Read the model definition and answer for the solid it produces. Units are mm, in the model's axes. Face numbers are marked on the shaded views. A direction names the side the tool comes from. Give positions to 0.01 mm unless a question says otherwise; leave off trailing zeros. Order: outer loops, then holes, each group sorted by start corner. A loop starts at its lowest first (then second) coordinate and runs counter-clockwise, first axis right, second up. Notation, with made-up numbers: (55, -5) - (88, -5) arc R19 ccw to (88, 5) - close; hole circle Ø1 at (-9.5, 76). An arc over 180 degrees is marked (long way). Use a Markdown table: item, result. Add a question column.
1. A cutting plane is placed at C-C on z = -17. Determine the outline of the cut face in (x, y).
2. A cutting plane is placed at B-B on y = 34.29. Determine the outline of the cut face in (x, z), and give its area (3 significant figures).
3. A cutting plane is placed at A-A on x = -21.59. Determine the outline of the cut face in (y, z).
4. Consider L1, parallel to Z at x = -21.59, y = 1.2; L2, parallel to X at y = 15.5, z = -8; L3, parallel to Y at x = -18.5, z = -25. Determine where each line is inside the solid, lowest interval first.
5. Which of the six approach directions +Z, -Z, +X, -X, +Y, -Y give full straight-line access (tool end or side, diameter ignored) to the marked faces 1 and 2?
6. Flat-ended cylindrical pins translate along their axes: P1, Ø4.5, axis at x = -21.59, z = -15.875, coming from the +Y side; P2, Ø1, axis at y = 28.5, z = -7, coming from the -X side; P3, Ø9, axis at x = -17, z = -10, coming from the +Y side. Find the tip coordinate at first contact, or state that the pin passes through.
7. A cutting plane is placed at D-D on z = -4. Determine the outline of the cut face in (x, y).
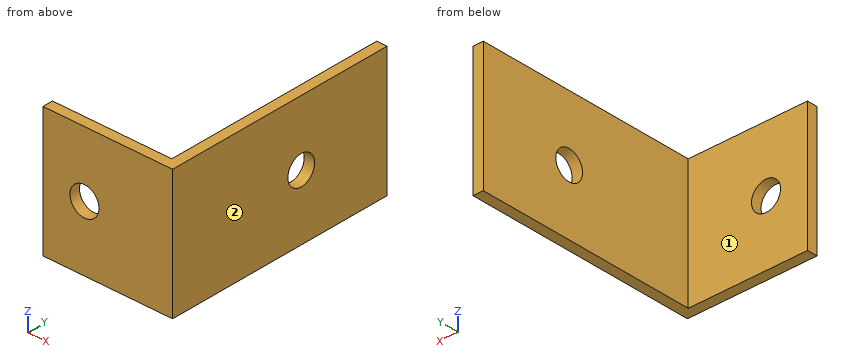
Autodesk Inventor part; units mm, degrees
ref_plane "YZ Plane" through (0, 0, 0) normal (1, 0, 0) x (0, 1, 0)
ref_plane "XZ Plane" through (0, 0, 0) normal (0, 1, 0) x (-1, 0, 0)
ref_plane "XY Plane" through (0, 0, 0) normal (0, 0, 1) x (1, 0, 0)
sketch "Sketch1" plane through (0, 0, 0) normal (0, 1, 0) x (-1, 0, 0)
  line L0 (0, 0) -> (31.75, 0)
  line L1 (31.75, 0) -> (31.75, -31.75)
  line L2 (31.75, -31.75) -> (0, -31.75)
  line L3 (0, -31.75) -> (0, 0)
  dimension "d0" = 31.75
  dimension "d1" = 31.75
extrude "Extrusion1" add sketch "Sketch1" along normal blind 2.54
sketch "Sketch2" plane through (0, 2.54, 0) normal (0, 1, 0) x (1, 0, 0)
  line L0 (0, 31.75) -> (-31.75, 31.75)
  line L1 (0, 0) -> (-2.54, 0)
  line L2 (-2.54, 0) -> (-2.54, 31.75)
  line L3 (-2.54, 31.75) -> (0, 31.75)
  line L4 (0, 31.75) -> (0, 0)
  dimension "d4" = 2.54
extrude "Extrusion2" add sketch "Sketch2" along normal blind 54.61
sketch "Sketch3" plane through (0, 2.54, 0) normal (0, 1, 0) x (1, 0, 0)
  line L0 (-2.54, 0) -> (-2.54, 31.75)
  line L1 (-2.54, 31.75) -> (-31.75, 31.75)
  line L2 (-31.75, 31.75) -> (-31.75, 0)
  line L3 (-31.75, 0) -> (-2.54, 0)
  point P0 (0, 0)
  point P1 (-21.59, 15.875)
  dimension "d7" = 15.875
  dimension "d8" = 19.05
hole "Hole1" at (-21.59, 2.54, -15.875) direction (0, -1, 0) diameter 7.112 end through all
sketch "Sketch4" plane through (-2.54, 2.54, -31.75) normal (-1, 0, 0) x (0, 0, 1)
  line L0 (31.75, 0) -> (0, 0)
  line L1 (31.75, 0) -> (31.75, 54.61)
  line L2 (0, 54.61) -> (31.75, 54.61)
  line L3 (0, 0) -> (0, 54.61)
  point P0 (31.75, -2.54)
  point P1 (15.875, 31.75)
  dimension "d16" = 15.875
  dimension "d17" = 31.75
hole "Hole2" at (-2.54, 34.29, -15.875) direction (1, 0, 0) diameter 7.112 end through all
properties part number "090001-1"
Output values:
| question | item | result |
|---|---|---|
| 1 | outline | (-31.75, 0) - (-24.96, 0) - (-24.96, 2.54) - (-31.75, 2.54) - close; (-18.22, 0) - (0, 0) - (0, 30.92) - (-2.54, 30.92) - (-2.54, 2.54) - (-18.22, 2.54) - close; (-2.54, 37.66) - (0, 37.66) - (0, 57.15) - (-2.54, 57.15) - close |
| 2 | outline | (-2.54, -31.75) - (0, -31.75) - (0, -19.43) - (-2.54, -19.43) - close; (-2.54, -12.32) - (0, -12.32) - (0, 0) - (-2.54, 0) - close |
| 2 | area | 62.6 mm² |
| 3 | outline | (0, -31.75) - (2.54, -31.75) - (2.54, -19.43) - (0, -19.43) - close; (0, -12.32) - (2.54, -12.32) - (2.54, 0) - (0, 0) - close |
| 4 | L1 | -31.75 to -19.43, -12.32 to 0 |
| 4 | L2 | -2.54 to 0 |
| 4 | L3 | 0 to 2.54 |
| 5 | face 1 | +Z, -Z, -X, +Y |
| 5 | face 2 | +Z, -Z, +X, +Y, -Y |
| 6 | P1 | through |
| 6 | P2 | x = -2.54 |
| 6 | P3 | y = 2.54 |
| 7 | outline | (-31.75, 0) - (0, 0) - (0, 57.15) - (-2.54, 57.15) - (-2.54, 2.54) - (-31.75, 2.54) - close |
